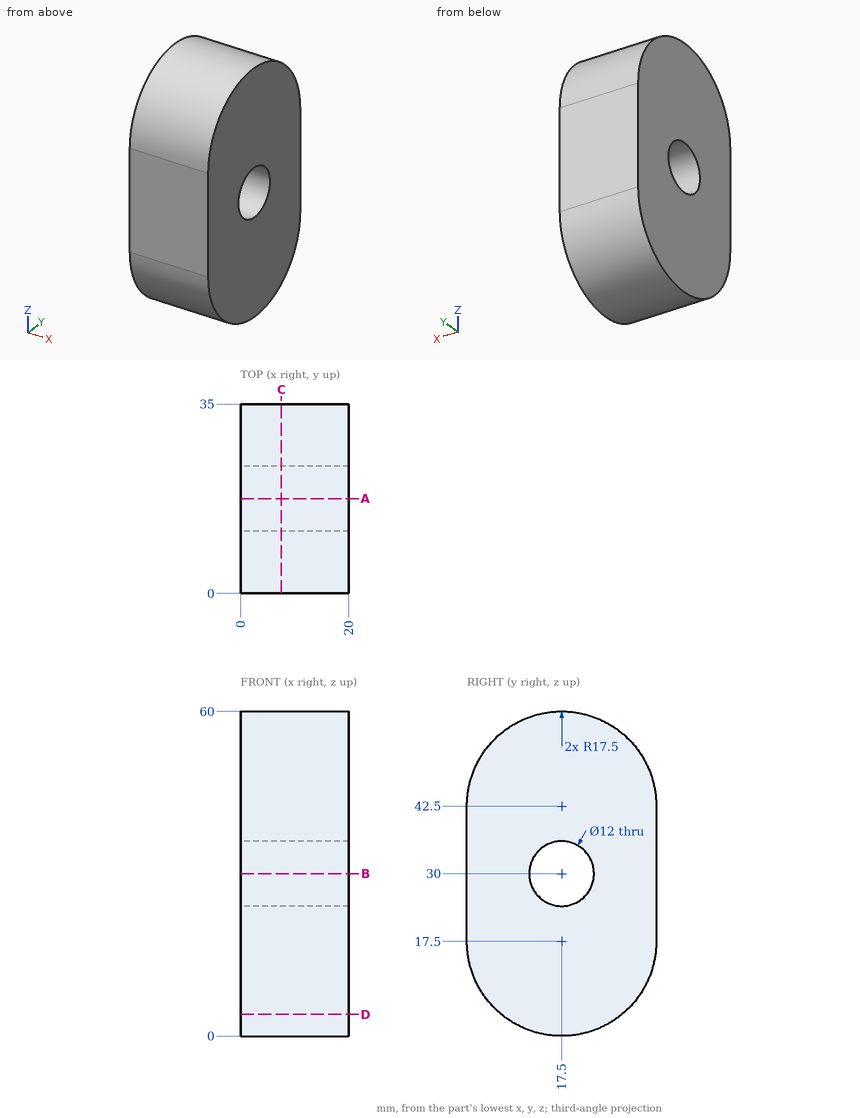
For this review, use the dimensioned drawing (mm, ordinates from the lowest corner) and the shaded views. Coordinates: 2 decimals unless noted, no trailing zeros. Loops run counter-clockwise (first coordinate to the right, second up) from the corner with the lowest first, then second, coordinate; pieces in that order, holes last. Notation, with made-up numbers: (24, 50) -> (72, 50) arc R32 ccw to (72, 89) -> close; hole circle Ø2 at (-4.5, 58). An arc over 180 degrees is marked (long way). Use a Markdown table: item, result. Add a question column.
1. Add section B-B on z = 30. Write out the cut boundary in (x, y).
2. Add section D-D on z = 4. Write out the cut boundary in (x, y).
3. Add section A-A on y = 17.5. Write out the cut boundary in (x, z).
4. To check wall thickness, follow line 1 (Y direction, x = 8.75, z = 30); line 2 (Z direction, x = 3.5, y = 13); line 3 (Y direction, x = 2.75, z = 28.5). State the ranges of each line that lie inside material, in increasing order.
5. Add section C-C on x = 7.5. Write out the cut boundary in (y, z).
6. Clearance check with flat-ended pins moving along their axes: pin 1 Ø4 at (x, z) = (4.5, 32) entering from -Y; pin 2 Ø3 at (x, z) = (11.5, 51) entering from -Y; pin 3 Ø8 at (x, y) = (12, 7.5) entering from -Z. State where each tip first meets the part, or that it passes through.
Returned:
| question | item | result |
|---|---|---|
| 1 | outline | (0, 0) -> (20, 0) -> (20, 11.5) -> (0, 11.5) -> close; (0, 23.5) -> (20, 23.5) -> (20, 35) -> (0, 35) -> close |
| 2 | outline | (0, 6.36) -> (20, 6.36) -> (20, 28.64) -> (0, 28.64) -> close |
| 3 | outline | (0, 0) -> (20, 0) -> (20, 24) -> (0, 24) -> close; (0, 36) -> (20, 36) -> (20, 60) -> (0, 60) -> close |
| 4 | line 1 | y = 0 to 11.5, 23.5 to 35 |
| 4 | line 2 | z = 0.59 to 26.03, 33.97 to 59.41 |
| 4 | line 3 | y = 0 to 11.69, 23.31 to 35 |
| 5 | outline | (0, 17.5) arc R17.5 ccw to (35, 17.5) -> (35, 42.5) arc R17.5 ccw to (0, 42.5) -> close; hole circle Ø12 at (17.5, 30) |
| 6 | pin 1 | stops at y = 0 |
| 6 | pin 2 | stops at y = 1.46 |
| 6 | pin 3 | stops at z = 1.06 |
